Part print with two shaded views. Sizes in mm from the minimum x, y, z corner. A direction names the side the tool comes from. Round coordinates to 2 decimals unless told otherwise and drop trailing zeros. Order: outer loops, then holes, each group sorted by start corner. A loop starts at its lowest first (then second) coordinate and runs counter-clockwise, first axis right, second up. Notation, with made-up numbers: M 44,81.25 L 86,81.25 A8 ccw 86,95.25 Z; hole C 50.25,22 d5. An arc over 180 degrees is marked long. Answer as a JSON object with one key per item and string values.
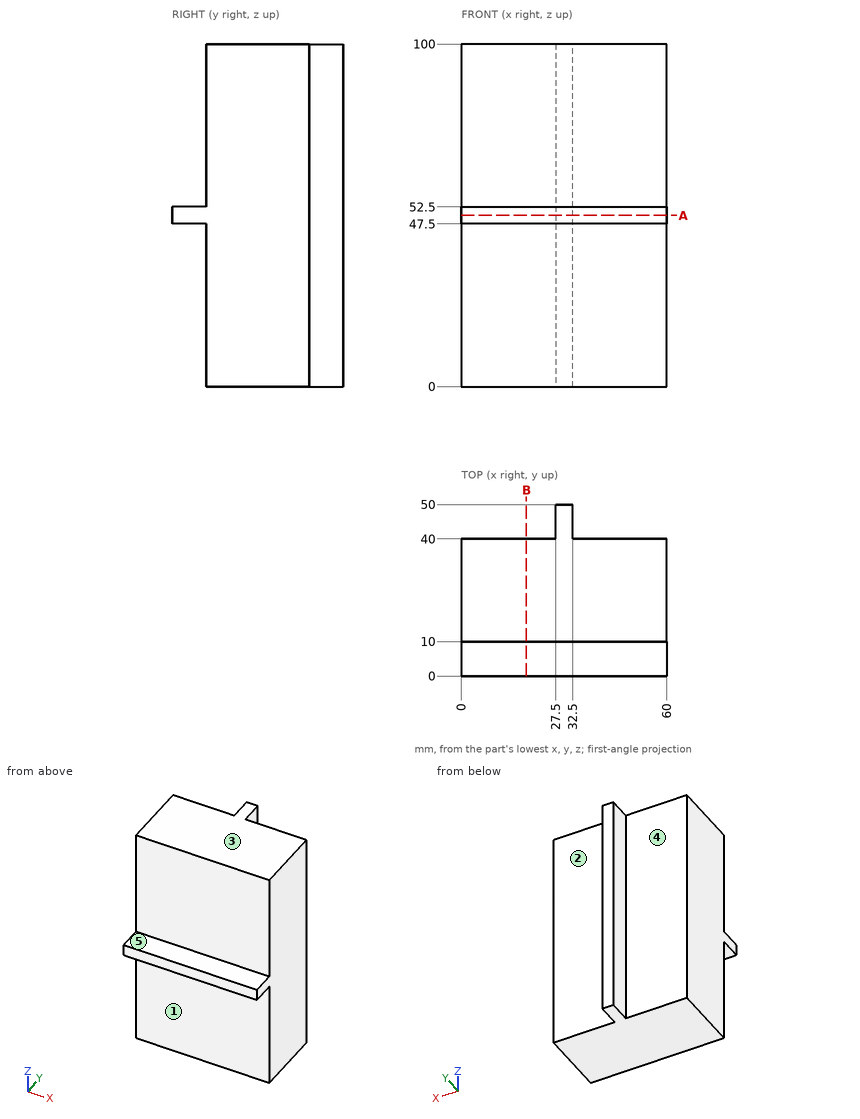
Item 1: Saw through at A-A on z = 50. List the corners of the cut face in (x, y), and give its area (3 significant figures).
Worked answers:
{"outline": "M 0,0 L 60,0 L 60,40 L 32.5,40 L 32.5,50 L 27.5,50 L 27.5,40 L 0,40 Z", "area": "2,450 mm2"}
Item 2: Drop flat-ended pins along their axis: pin 1 Ø14 at (x, z) = (8, 71.5) entering from +Y; pin 2 Ø24 at (x, z) = (34, 87.5) entering from -Y; pin 3 Ø5 at (y, z) = (47, 34) entering from +X. Give the stop position or say it passes through.
Worked answers:
{"pin 1": "stops at y = 40", "pin 2": "stops at y = 10", "pin 3": "stops at x = 32.5"}
Item 3: 3-axis set-ups, long thin cutter, end or side, ignore diameter. For the marked faces 1, 2, 3, 4 and 5: which of +Z, -Z, +X, -X, +Y, -Y reach the whole face in a straight line?
Worked answers:
{"face 1": "-Z, +X, -X, -Y", "face 2": "+Z, -Z, +X, +Y", "face 3": "+Z, +X, -X, +Y, -Y", "face 4": "+Z, -Z, -X, +Y", "face 5": "+Z, +X, -X, -Y"}
Item 4: Saw through at B-B on x = 19. List the corners of the cut face in (y, z), and give its area (3 significant figures).
Worked answers:
{"outline": "M 0,47.5 L 10,47.5 L 10,0 L 40,0 L 40,100 L 10,100 L 10,52.5 L 0,52.5 Z", "area": "3,050 mm2"}
Item 5: Wall check: line 1 along Y through (x, z) = (45, 70); line 2 along X through (y, z) = (40.5, 60.5); line 3 along Z through (x, y) = (21.5, 6). Give the ranges that are in metal, low to high. Write a range as [from, to].
Worked answers:
{"line 1": "y = [10, 40]", "line 2": "x = [27.5, 32.5]", "line 3": "z = [47.5, 52.5]"}
